Geometry check sheet. Reference: the model listing, model coordinates, mm. Face numbers are marked on the shaded views. A direction names the side the tool comes from. Give positions to 0.01 mm unless a question says otherwise; leave off trailing zeros. Loops run counter-clockwise (first coordinate to the right, second up) from the corner with the lowest first, then second, coordinate; pieces in that order, holes last. Notation, with made-up numbers: (47.5, -3.75) -> (83.5, -3.75) arc R10 ccw to (83.5, 8.25) -> close; hole circle Ø1 at (-20, 84). An arc over 180 degrees is marked (long way). Answer in a Markdown table with one row per item. Add a question column.
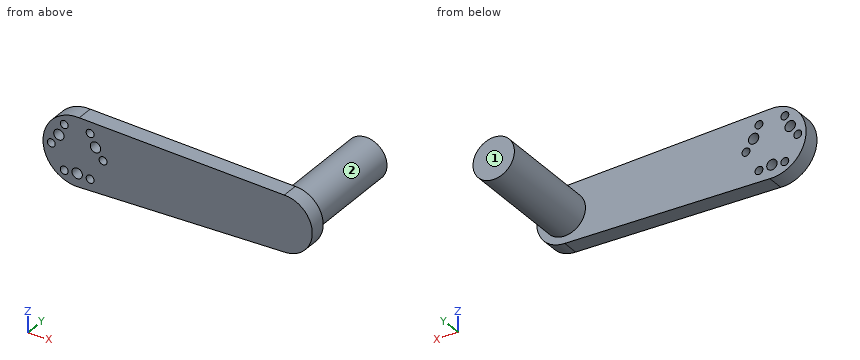
```python
from build123d import *

# Parameters (mm, degrees)
SKETCH_1_R               = 16.5
EXTRUDE_1_DEPTH          = 8
CUT_EXTRUDE_1_DEPTH      = 25.667792767
CUT_EXTRUDE_1_DEPTH_BACK = 25.667792767
SKETCH_4_R               = 2.5
SKETCH_4_R_2             = 1.9
SKETCH_1_3_R             = 10
EXTRUDE_2_DEPTH          = 8
SKETCH_1_4_R             = 10
EXTRUDE_3_DEPTH          = 60


with BuildPart() as part:
    # Sketch 1 → Extrude 1 (new body)
    with BuildSketch(Plane(origin=(0, 0, 0), x_dir=(1, 0, 0), z_dir=(0, 1, 0))):
        with Locations(Location((0, 0, 0), (0, 0, 270))):
            Circle(SKETCH_1_R)
    extrude(amount=EXTRUDE_1_DEPTH)

    # Sketch 4 → Cut-Extrude 1 (cut, two sides: drawn at the far end of the back side and taken through both)
    with BuildSketch(Plane(origin=(0, 8, 0), x_dir=(1, 0, 0), z_dir=(0, 1, 0)).offset(-CUT_EXTRUDE_1_DEPTH_BACK)):
        with Locations(Location((0, 10.2, 0), (0, 0, 270))):
            Circle(SKETCH_4_R)
        with Locations(Location((-6.25, 10.825317547, 0), (0, 0, 270))):
            Circle(SKETCH_4_R_2)
        with Locations(Location((6.25, 10.825317547, 0), (0, 0, 270))):
            Circle(SKETCH_4_R_2)
        with Locations(Location((12.5, 0, 0), (0, 0, 270))):
            Circle(SKETCH_4_R_2)
        with Locations(Location((6.25, -10.825317547, 0), (0, 0, 270))):
            Circle(SKETCH_4_R_2)
        with Locations(Location((-6.25, -10.825317547, 0), (0, 0, 270))):
            Circle(SKETCH_4_R_2)
        with Locations(Location((-12.5, 0, 0), (0, 0, 270))):
            Circle(SKETCH_4_R_2)
        with Locations(Location((8.833459119, -5.1, 0), (0, 0, 270))):
            Circle(SKETCH_4_R)
        with Locations(Location((-8.833459119, -5.1, 0), (0, 0, 270))):
            Circle(SKETCH_4_R)
    extrude(amount=CUT_EXTRUDE_1_DEPTH + CUT_EXTRUDE_1_DEPTH_BACK, mode=Mode.SUBTRACT)

    # Sketch 1_3 → Extrude 2 (add)
    with BuildSketch(Plane(origin=(0, 0, 0), x_dir=(1, 0, 0), z_dir=(0, 1, 0))):
        with BuildLine():
            ThreePointArc((0.989109801, 16.470326706), (16.5, 0), (0.989109801, -16.470326706))
            Line((0.989109801, -16.470326706), (100, -13.5))
            ThreePointArc((100, -13.5), (113.5, 0), (100, 13.5))
            Line((100, 13.5), (0.989109801, 16.470326706))
        make_face()
        with Locations(Location((100, 0, 0), (0, 0, 270))):
            Circle(SKETCH_1_3_R, mode=Mode.SUBTRACT)
    extrude(amount=EXTRUDE_2_DEPTH)

    # Sketch 1_4 → Extrude 3 (add)
    with BuildSketch(Plane(origin=(0, 0, 0), x_dir=(1, 0, 0), z_dir=(0, 1, 0))):
        with Locations(Location((100, 0, 0), (0, 0, 270))):
            Circle(SKETCH_1_4_R)
    extrude(amount=EXTRUDE_3_DEPTH)


solid = part.part
```
1. Access from +Z, -Z, +X, -X, +Y, -Y to the whole of each face (thin tool, end or side, straight path). Record for the marked faces 1 and 2.
2. Gauge pin test, flat ends, axial feed: pin 1 Ø16.5 at (x, z) = (49, 6) entering from +Y; pin 2 Ø10 at (y, z) = (31, -5) entering from +X; pin 3 Ø6 at (x, z) = (-6.25, -10.83) entering from -Y; pin 4 Ø1 at (y, z) = (49.5, 5.5) entering from +X. Record the tip position at first contact, or that the pin passes through.
3. Sectioned sample at C-C (x = 104.5). Enter the section's corners in (y, z).
4. Material ranges on L1, parallel to X at y = 3.5, z = -10.5; L2, parallel to Z at x = -6, y = 5; L3, parallel to Y at x = 31, z = 12, recorded low to high. Write a range as from..to.
5. Sectioned sample at A-A (z = 0). Enter the section's corners in (x, y), plus the area to 3 significant figures.
6. Sectioned sample at B-B (y = 28). Enter the section's corners in (x, z).
Response:
| question | item | result |
|---|---|---|
| 1 | face 1 | +Z, -Z, +X, -X, +Y |
| 1 | face 2 | +Y |
| 2 | pin 1 | stops at y = 8 |
| 2 | pin 2 | stops at x = 110 |
| 2 | pin 3 | stops at y = 0 |
| 2 | pin 4 | stops at x = 108.66 |
| 3 | outline | (0, -12.73) -> (8, -12.73) -> (8, -8.93) -> (60, -8.93) -> (60, 8.93) -> (8, 8.93) -> (8, 12.73) -> (0, 12.73) -> close |
| 4 | L1 | x = -12.73..-8.12, -4.38..-2.48, 2.48..4.38, 8.12..108.49 |
| 4 | L2 | z = -15.37..-12.71, -8.94..8.94, 12.71..15.37 |
| 4 | L3 | y = 0..8 |
| 5 | outline | (-16.5, 0) -> (-14.4, 0) -> (-14.4, 8) -> (-16.5, 8) -> close; (-10.6, 0) -> (10.6, 0) -> (10.6, 8) -> (-10.6, 8) -> close; (14.4, 0) -> (113.5, 0) -> (113.5, 8) -> (110, 8) -> (110, 60) -> (90, 60) -> (90, 8) -> (14.4, 8) -> close |
| 5 | area | 2,020 mm2 |
| 6 | outline | circle Ø20 at (100, 0) |
